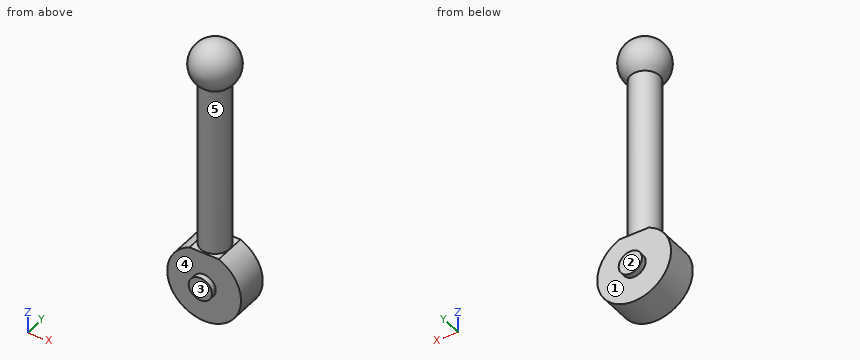
from build123d import *

# Parameters (mm, degrees)
F0_R     = 2.16
F1_DEPTH = 1.9
F3_R     = 0.68
F4_DEPTH = 0.33
F5_R     = 0.68
F6_DEPTH = 0.33
F7_DEPTH = 25
F8_R     = 0.84
F9_DEPTH = 11


with BuildPart() as f1:
    # F0 (on Front) → F1 (new body)
    with BuildSketch(Plane.XZ):
        Circle(F0_R)
    extrude(amount=F1_DEPTH)

    # F3 (on face) → F4 (join)
    with BuildSketch(Plane.XZ.offset(1.9)):
        Circle(F3_R)
    extrude(amount=F4_DEPTH)

    # F5 (on face) → F6 (join)
    with BuildSketch(Plane(origin=(0, 0, 0), x_dir=(-1, 0, 0), z_dir=(0, 1, 0))):
        Circle(F5_R)
    extrude(amount=F6_DEPTH)

    # F2 (on face) → F7 (cut)
    with BuildSketch(Plane.XZ.offset(1.9)):
        with BuildLine():
            ThreePointArc((0.854606, 1.983746), (0, 2.16), (-0.854606, 1.983746))
            Line((-0.854606, 1.983746), (0.854606, 1.983746))
        make_face()
    extrude(amount=-F7_DEPTH, mode=Mode.SUBTRACT)

    # F8 (on face) → F9 (join)
    with BuildSketch(Plane.XY.offset(1.983746)):
        with Locations((0, -0.95)):
            Circle(F8_R)
    extrude(amount=F9_DEPTH)

    # F10 (on face) → F11 (revolve)
    with BuildSketch(Plane.XY.offset(12.983746)):
        with BuildLine():
            Line((0, -2.305), (0, 0.405))
            ThreePointArc((0, 0.405), (-1.355, -0.95), (0, -2.305))
        make_face()
        with BuildLine():
            Line((0, -0.11), (0, 0.405))
            ThreePointArc((0, 0.405), (-1.355, -0.95), (0, -2.305))
            Line((0, -2.305), (0, -1.79))
            ThreePointArc((0, -1.79), (-0.84, -0.95), (0, -0.11))
        make_face()
    revolve(axis=Axis((0, -0.95, 12.983746), (0, -1, 0)))


solid = f1.part
Part model, mm, in its own coordinate system. Face numbers are marked on the shaded views. A direction names the side the tool comes from. Coordinates: 2 decimals unless noted, no trailing zeros. Loops run counter-clockwise (first coordinate to the right, second up) from the corner with the lowest first, then second, coordinate; pieces in that order, holes last. Notation, with made-up numbers: (47, 37.25) -> (98, 37.25) arc R12 ccw to (98, 51.25) -> close; hole circle Ø2 at (88, 88). An arc over 180 degrees is marked (long way). Use a Markdown table: item, result. Add a question column.
Item 1: Pull direction Z, two halves, no side cores. Call the marked faces 1 and 2: +Z half, -Z half, draft (parallel to the pull), parting line (faces both ways), or undercut.
Item 2: Probe probe 1 along Y at (x, z) = (0.2, 0.5); probe 2 along Y at (x, z) = (-0.75, 0.5); probe 3 along Z at (x, y) = (0.55, -0.2). List the from-to ranges inside material, lowest first.
Item 3: Which spindle directions (+Z, -Z, +X, -X, +Y, -Y) get a long thin tool onto all of the face, cutting with end or side? Do the marked faces 3, 4 and 5. Say none if no direction does.
Item 4: Band-saw the part on C-C on y = -0.95. Write the cut outline in (x, z) (3 decimals), plus the area to 3 significant figures.
Item 5: Flat gauge pins, fed straight in: P1, Ø1.5, axis at y = -1.5, z = 2.5, coming from the -X side; P2, Ø1.2, axis at x = 0, z = -0.5, coming from the -Y side; P3, Ø0.7, axis at x = 0.5, z = 0, coming from the +Y side; P4, Ø1.4, axis at x = 0, y = -0.5, coming from the +Z side. Where does each tip first touch, or does it go through?
Item 6: Band-saw the part on D-D on x = -1.05. Write the cut outline in (y, z).
Item 7: Band-saw the part on B-B on x = 0. Write the cut outline in (y, z) (3 decimals).
Item 8: Band-saw the part on A-A on z = 0. Write the cut outline in (x, y).
Geometry says:
| question | item | result |
|---|---|---|
| 1 | face 1 | undercut |
| 1 | face 2 | draft |
| 2 | probe 1 | -2.23 to 0.33 |
| 2 | probe 2 | -1.9 to 0 |
| 2 | probe 3 | -2.09 to 1.98, 12 to 13.97 |
| 3 | face 3 | -Z, +X, -X, -Y |
| 3 | face 4 | -Y |
| 3 | face 5 | none |
| 4 | outline | (-0.855, 1.984) arc R2.16 ccw (long way) to (0.855, 1.984) -> (0.84, 1.984) -> (0.84, 11.921) arc R1.355 ccw (long way) to (-0.84, 11.921) -> (-0.84, 1.984) -> close |
| 4 | area | 36.6 mm² |
| 5 | P1 | x = -1.27 |
| 5 | P2 | y = -2.23 |
| 5 | P3 | y = 0.33 |
| 5 | P4 | z = 14.34 |
| 6 | outline | (-1.9, -1.89) -> (0, -1.89) -> (0, 1.89) -> (-1.9, 1.89) -> close; circle Ø1.71 at (-0.95, 12.98) |
| 7 | outline | (-2.23, -0.68) -> (-1.9, -0.68) -> (-1.9, -2.16) -> (0, -2.16) -> (0, -0.68) -> (0.33, -0.68) -> (0.33, 0.68) -> (0, 0.68) -> (0, 1.984) -> (-0.11, 1.984) -> (-0.11, 11.921) arc R1.355 ccw (long way) to (-1.79, 11.921) -> (-1.79, 1.984) -> (-1.9, 1.984) -> (-1.9, 0.68) -> (-2.23, 0.68) -> close |
| 8 | outline | (-2.16, -1.9) -> (-0.68, -1.9) -> (-0.68, -2.23) -> (0.68, -2.23) -> (0.68, -1.9) -> (2.16, -1.9) -> (2.16, 0) -> (0.68, 0) -> (0.68, 0.33) -> (-0.68, 0.33) -> (-0.68, 0) -> (-2.16, 0) -> close |
